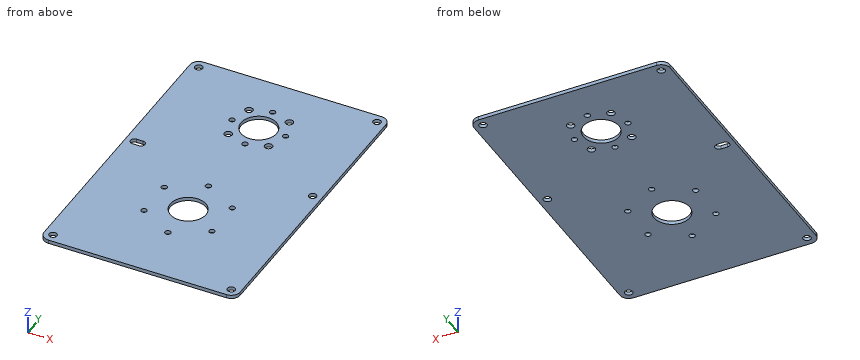
Autodesk Inventor part; units mm, degrees
ref_plane "YZ Plane" through (0, 0, 0) normal (1, 0, 0) x (0, 1, 0)
ref_plane "XZ Plane" through (0, 0, 0) normal (0, 1, 0) x (-1, 0, 0)
ref_plane "XY Plane" through (0, 0, 0) normal (0, 0, 1) x (1, 0, 0)
sketch "スケッチ1" plane through (0, 0, 0) normal (0, 0, 1) x (1, 0, 0)
  line L0 (55, -93.4) -> (-55, -93.4)
  line L1 (-55, -93.4) -> (-55, 75)
  line L2 (-55, 75) -> (55, 75)
  line L3 (55, 75) -> (55, -93.4)
  line L4 (55, -93.4) -> (-55, 75) construction
  line L5 (-55, -93.4) -> (55, 75) construction
  point P0 (0, 0)
  point P1 (0, -9.2)
  point P2 (0, -9.2)
  dimension "d50" = 93.4
  dimension "d51" = 110
  dimension "d52" = 75
extrude "プレート1" add sketch "スケッチ1" along normal blind 2
sketch "スケッチ3" plane through (0, 0, 2) normal (0, 0, 1) x (1, 0, 0)
  circle A0 centre (0, 38.4) radius 10
  circle A1 centre (0, -38.4) radius 10
  point P0 (0, 0)
  dimension "d22" = 20
  dimension "d53" = 20
  dimension "d55" = 76.8
  dimension "d56" = 38.4
extrude "押し出し1" cut sketch "スケッチ3" against normal blind 10 contours A0
sketch "スケッチ2" plane through (0, 0, 2) normal (0, 0, 1) x (1, 0, 0)
  circle A0 centre (0, 38.4) radius 15 construction
  circle A1 centre (0, -38.4) radius 22
  point P0 (0, 0)
  point P1 (0, 53.4)
  point P2 (-15, 38.4)
  point P3 (0, 23.4)
  point P4 (15, 38.4)
  point P5 (0, -16.4)
  point P6 (-19.0526, -27.4)
  point P7 (-19.0526, -49.4)
  point P8 (0, -60.4)
  point P9 (19.0526, -49.4)
  point P10 (19.0526, -27.4)
  dimension "d3" = 30
  dimension "d8" = 44
  dimension "d6" = 360
  dimension "d11" = 360
  dimension "d13" = 76.8
  dimension "d14" = 38.4
hole "穴1" at (0, 53.4, 2) at (-15, 38.4, 2) at (0, 23.4, 2) at (15, 38.4, 2) at (0, -16.4, 2) at (-19.0526, -27.4, 2) at (-19.0526, -49.4, 2) at (0, -60.4, 2) at (19.0526, -27.4, 2) at (19.0526, -49.4, 2) direction (0, 0, -1) diameter 3.2 end through all
sketch "スケッチ4" plane through (0, 0, 2) normal (0, 0, 1) x (1, 0, 0)
  line L0 (55, -93.4) -> (-55, -93.4)
  line L1 (-55, -93.4) -> (-55, 75)
  line L2 (55, 75) -> (55, -93.4)
  line L3 (-55, 75) -> (55, 75)
  line L4 (-50, 70) -> (-50, -88.4)
  line L5 (-50, -88.4) -> (50, -88.4)
  line L6 (50, -88.4) -> (50, 70)
  line L7 (50, 70) -> (-50, 70)
  point P0 (-50, 0)
  point P1 (50, 0)
  point P2 (0, 0)
  dimension "d57" = 5
hole "穴2" at (-50, -88.4, 2) at (50, -88.4, 2) at (50, 70, 2) at (-50, 70, 2) at (-50, 0, 2) at (50, 0, 2) direction (0, 0, -1) diameter 4.3 end through all
fillet "コーナーR1" radius 5 4 edges at (-55, -93.4, 1) (55, -93.4, 1) (55, 75, 1) (-55, 75, 1)
sketch "スケッチ5" plane through (0, 0, 2) normal (0, 0, 1) x (1, 0, 0)
  circle A0 centre (0, -38.4) radius 10
  point P0 (0, 0)
  dimension "d35" = 20
extrude "押し出し2" cut sketch "スケッチ5" against normal blind 10
sketch "スケッチ6" plane through (0, 0, 2) normal (0, 0, 1) x (1, 0, 0)
  circle A0 centre (0, 38.4) radius 10
  circle A1 centre (0, 38.4) radius 16
  point P0 (0, 0)
  point P1 (-11.3137, 49.7137)
  point P2 (-11.3137, 27.0863)
  point P3 (11.3137, 27.0863)
  point P4 (11.3137, 49.7137)
  dimension "d38" = 32
  dimension "d41" = 360
hole "穴3" at (-11.3137, 49.7137, 2) at (-11.3137, 27.0863, 2) at (11.3137, 27.0863, 2) at (11.3137, 49.7137, 2) direction (0, 0, -1) diameter 4.3 end through all
sketch "スケッチ7" plane through (0, 0, 2) normal (0, 0, 1) x (1, 0, 0)
  line L0 (-46.2, 0) -> (-50, 0) construction
  line L1 (-46.2, 2.15) -> (-50, 2.15)
  line L2 (-50, -2.15) -> (-46.2, -2.15)
  arc A0 (-46.2, -2.15) -> (-46.2, 2.15) centre (-46.2, 0) ccw
  arc A1 (-50, 2.15) -> (-50, -2.15) centre (-50, 0) ccw
  circle A2 centre (-50, 0) radius 2.15
  point P0 (0, 0)
  point P1 (-48.1, 0)
  dimension "d58" = 48.1
extrude "押し出し3" cut sketch "スケッチ7" against normal blind 10
equation "\"d20\" = Thickness"
equation "\"d2\" = Thickness"
equation "\"BendRadius\" = Thickness"
equation "\"BendReliefWidth\" = Thickness"
equation "\"BendReliefDepth\" = 0.5 * Thickness"
equation "\"CornerReliefSize\" = 4 * Thickness"
equation "\"MinimumRemnant\" = 2 * Thickness"
equation "\"TransitionRadius\" = BendRadius"
equation "\"JacobiRadiusSize\" = BendRadius"
equation "\"GapSize\" = Thickness"
properties part number "carbonplate1" material "CFRP"
Source: CAD feature listing. Evaluate the final solid. Frame: model axes, mm. Coordinates: 2 decimals unless noted, no trailing zeros. Order: outer loops, then holes, each group sorted by start corner. A loop starts at its lowest first (then second) coordinate and runs counter-clockwise, first axis right, second up. Notation, with made-up numbers: M 65,78.25 L 106,78.25 A17 ccw 106,102.25 Z; hole C 52,-27.75 d4. An arc over 180 degrees is marked long. Write each question's results on one line, items separated by ' | '. Start each with the question number.
1. Material intervals for L1, parallel to X at y = -27.4, z = 1.05; L2, parallel to X at y = 39, z = 0.1; L3, parallel to Y at x = 15, z = 1.2, sorted ascending.
2. Pin query (flat end, axial travel): pin 1 (3 mm diameter, centred on x = 25, y = -52, fed in from -Z). Return the tip coordinate at first contact, or that it passes through.
3. Section D-D, the plane z = 0.3. State how many separate pieces and enclosed holes the cut face has, then the cut area to 3 significant figures.
4. Section C-C, the plane y = -36. Return the cut outline in (x, z).
5. Section B-B, the plane x = -4.5. Return the cut outline in (y, z), then the cut area to 3 significant figures.
6. Section A-A, the plane y = 0. Return the cut outline in (x, z).
Solution:
1) L1: -55 to -20.65, -17.45 to 17.45, 20.65 to 55 | L2: -55 to -16.48, -13.52 to -9.98, 9.98 to 13.52, 16.48 to 55 | L3: -93.4 to 36.8, 40 to 75
2) pin 1: z = 0
3) separate pieces: 1 | enclosed holes: 22 | area: 17,600 mm²
4) outline: M -55,0 L -9.71,0 L -9.71,2 L -55,2 Z; M 9.71,0 L 55,0 L 55,2 L 9.71,2 Z
5) outline: M -93.4,0 L -47.33,0 L -47.33,2 L -93.4,2 Z; M -29.47,0 L 29.47,0 L 29.47,2 L -29.47,2 Z; M 47.33,0 L 75,0 L 75,2 L 47.33,2 Z | area: 265 mm²
6) outline: M -55,0 L -52.15,0 L -52.15,2 L -55,2 Z; M -44.05,0 L 47.85,0 L 47.85,2 L -44.05,2 Z; M 52.15,0 L 55,0 L 55,2 L 52.15,2 Z
